from build123d import *

# Parameters (mm, degrees)
SKETCH1_R      = 9.25
SKETCH1_R_2    = 33.475
EXTRUDE2_DEPTH = 1.2


with BuildPart() as part:
    # Sketch1 → Extrude2 (new body)
    with BuildSketch(Plane.XY):
        with BuildLine():
            Line((-26.875, -52.5), (26.875, -52.5))
            ThreePointArc((26.875, -52.5), (35.790865916, -49.562642122), (41.214853301, -41.900977995))
            ThreePointArc((41.214853301, -41.900977995), (47.5, 0), (41.214853301, 41.900977995))
            ThreePointArc((41.214853301, 41.900977995), (35.790865916, 49.562642122), (26.875, 52.5))
            Line((26.875, 52.5), (-26.875, 52.5))
            ThreePointArc((-26.875, 52.5), (-35.790865916, 49.562642122), (-41.214853301, 41.900977995))
            ThreePointArc((-41.214853301, 41.900977995), (-47.5, 0), (-41.214853301, -41.900977995))
            ThreePointArc((-41.214853301, -41.900977995), (-35.790865916, -49.562642122), (-26.875, -52.5))
        make_face()
        with Locations((-28, -38)):
            Circle(SKETCH1_R, mode=Mode.SUBTRACT)
        with Locations((28, -38)):
            Circle(SKETCH1_R, mode=Mode.SUBTRACT)
        with Locations((28, 38)):
            Circle(SKETCH1_R, mode=Mode.SUBTRACT)
        with Locations((-28, 38)):
            Circle(SKETCH1_R, mode=Mode.SUBTRACT)
        Circle(SKETCH1_R_2, mode=Mode.SUBTRACT)
    extrude(amount=EXTRUDE2_DEPTH)


solid = part.part
For this review, take the finished solid that the model builds, in its own axes (mm). Round coordinates to 2 decimals unless told otherwise and drop trailing zeros. Loops run counter-clockwise (first coordinate to the right, second up) from the corner with the lowest first, then second, coordinate; pieces in that order, holes last. Notation, with made-up numbers: (74, 66) - (79, 66) arc R16 cw to (79, 88) - close; hole circle Ø3 at (27.5, 69.25). An arc over 180 degrees is marked (long way). One line per item, written item: value. Start each with the question number.
Item 1: Take a section at C-C (y = 38). Give the boundary of the cut face in (x, z).
Item 2: The part is to be moulded in two halves that separate along Y. For faces 1 (the flat face through (-32, 12, 0)), 2 (the cylindrical face through (47.5, -0.6, 0.6)), 3 (the cylindrical face through (21.18, -31.75, 0.59)), say which applies: +Y half, -Y half, draft (parallel to the pull), parting line (faces both ways), or undercut.
Item 3: Take a section at A-A (y = 0). Give the boundary of the cut face in (x, z) (3 decimals), plus the area to 3 significant figures.
Item 4: Take a section at B-B (z = 1). State how many separate pieces and enclosed holes the cut face has, plus the area to 3 significant figures.
Item 5: Clearance check with a flat-ended pin moving along its axis: pin 1 Ø24 at (x, y) = (28, -38) entering from -Z. State where the tip first meets the part, or that it passes through.
Item 6: Take a section at D-D (x = -23). Give the boundary of the cut face in (y, z), plus the area to 3 significant figures.
Item 7: For L1, parallel to Y at x = 28, z = 0.4; L2, parallel to Y at x = 21, z = 0.65; L3, parallel to Y at x = -34.5, z = 0.7, list the stretches that pass through material, from the lowest coordinate up.
Answer below:
1. outline: (-42.35, 0) - (-37.25, 0) - (-37.25, 1.2) - (-42.35, 1.2) - close; (-18.75, 0) - (18.75, 0) - (18.75, 1.2) - (-18.75, 1.2) - close; (37.25, 0) - (42.35, 0) - (42.35, 1.2) - (37.25, 1.2) - close
2. face 1: draft
2. face 2: parting line
2. face 3: undercut
3. outline: (-47.5, 0) - (-33.475, 0) - (-33.475, 1.2) - (-47.5, 1.2) - close; (33.475, 0) - (47.5, 0) - (47.5, 1.2) - (33.475, 1.2) - close
3. area: 33.7 mm2
4. separate pieces: 1
4. enclosed holes: 5
4. area: 4,600 mm2
5. pin 1: stops at z = 0
6. outline: (-52.5, 0) - (-45.78, 0) - (-45.78, 1.2) - (-52.5, 1.2) - close; (-30.22, 0) - (-24.32, 0) - (-24.32, 1.2) - (-30.22, 1.2) - close; (24.32, 0) - (30.22, 0) - (30.22, 1.2) - (24.32, 1.2) - close; (45.78, 0) - (52.5, 0) - (52.5, 1.2) - (45.78, 1.2) - close
6. area: 30.3 mm2
7. L1: y = -52.46 to -47.25, -28.75 to -18.35, 18.35 to 28.75, 47.25 to 52.46
7. L2: y = -52.5 to -44.05, -31.95 to -26.07, 26.07 to 31.95, 44.05 to 52.5
7. L3: y = -50.42 to -44.58, -31.42 to 31.42, 44.58 to 50.42
